Work out the finished part from the listing and answer in its coordinate system (mm). Coordinates: 2 decimals unless noted, no trailing zeros. Order: outer loops, then holes, each group sorted by start corner. A loop starts at its lowest first (then second) coordinate and runs counter-clockwise, first axis right, second up. Notation, with made-up numbers: (5.25, 61.25) -> (60.25, 61.25) arc R34 ccw to (60.25, 100.25) -> close; hole circle Ø3 at (0.25, 58.5). An arc over 180 degrees is marked (long way). Use one line per item in the form item = value.
from build123d import *

# Parameters (mm, degrees)
SKETCH_1_W      = 63
SKETCH_1_H      = 42
SKETCH_1_R      = 4.5
SKETCH_1_W_2    = 10
SKETCH_1_W_3    = 42
SKETCH_1_R_2    = 1.6
SKETCH_1_W_4    = 5
EXTRUDE_1_DEPTH = 6
FILLET_1_R      = 5


with BuildPart() as part:
    # 草图1 → 凸台-拉伸1 (new body)
    # profile 1 of 7: a face of its own
    with BuildSketch(Plane.XY):
        with Locations((-109.5, 0)):
            Rectangle(SKETCH_1_W, SKETCH_1_H)
        with Locations((-132, 0)):
            Circle(SKETCH_1_R, mode=Mode.SUBTRACT)
    # profile 2 of 7: a face of its own
    with BuildSketch(Plane.XY):
        with BuildLine():
            Line((-73, 21), (-78, 21))
            Line((-78, 21), (-78, -21))
            Line((-78, -21), (-73, -21))
            Line((-73, -21), (-73, -17.019868415))
            ThreePointArc((-73, -17.019868415), (-74.1, -15.5), (-73, -13.980131585))
            Line((-73, -13.980131585), (-73, 13.980131585))
            ThreePointArc((-73, 13.980131585), (-74.1, 15.5), (-73, 17.019868415))
            Line((-73, 17.019868415), (-73, 21))
        make_face()
    # profile 3 of 7: a face of its own
    with BuildSketch(Plane.XY):
        with BuildLine():
            Line((-36, 21), (-73, 21))
            Line((-73, 21), (-73, 17.019868415))
            ThreePointArc((-73, 17.019868415), (-72.753190181, 17.079840097), (-72.5, 17.1))
            Line((-72.5, 17.1), (-67.5, 17.1))
            ThreePointArc((-67.5, 17.1), (-65.9, 15.5), (-67.5, 13.9))
            Line((-67.5, 13.9), (-72.5, 13.9))
            ThreePointArc((-72.5, 13.9), (-72.753190181, 13.920159903), (-73, 13.980131585))
            Line((-73, 13.980131585), (-73, -13.980131585))
            ThreePointArc((-73, -13.980131585), (-72.753190181, -13.920159903), (-72.5, -13.9))
            Line((-72.5, -13.9), (-67.5, -13.9))
            ThreePointArc((-67.5, -13.9), (-65.9, -15.5), (-67.5, -17.1))
            Line((-67.5, -17.1), (-72.5, -17.1))
            ThreePointArc((-72.5, -17.1), (-72.753190181, -17.079840097), (-73, -17.019868415))
            Line((-73, -17.019868415), (-73, -21))
            Line((-73, -21), (-36, -21))
            Line((-36, -21), (-36, -17.019868415))
            ThreePointArc((-36, -17.019868415), (-36.246809819, -17.079840097), (-36.5, -17.1))
            Line((-36.5, -17.1), (-41.5, -17.1))
            ThreePointArc((-41.5, -17.1), (-43.1, -15.5), (-41.5, -13.9))
            Line((-41.5, -13.9), (-36.5, -13.9))
            ThreePointArc((-36.5, -13.9), (-36.246809819, -13.920159903), (-36, -13.980131585))
            Line((-36, -13.980131585), (-36, 13.980131585))
            ThreePointArc((-36, 13.980131585), (-36.246809819, 13.920159903), (-36.5, 13.9))
            Line((-36.5, 13.9), (-41.5, 13.9))
            ThreePointArc((-41.5, 13.9), (-43.1, 15.5), (-41.5, 17.1))
            Line((-41.5, 17.1), (-36.5, 17.1))
            ThreePointArc((-36.5, 17.1), (-36.246809819, 17.079840097), (-36, 17.019868415))
            Line((-36, 17.019868415), (-36, 21))
        make_face()
        with BuildLine():
            ThreePointArc((-57, -2.5), (-59.5, 0), (-57, 2.5))
            Line((-57, 2.5), (-52, 2.5))
            ThreePointArc((-52, 2.5), (-49.5, 0), (-52, -2.5))
            Line((-52, -2.5), (-57, -2.5))
        make_face(mode=Mode.SUBTRACT)
    # profile 4 of 7: a face of its own
    with BuildSketch(Plane.XY):
        with BuildLine():
            Line((-31, 21), (-36, 21))
            Line((-36, 21), (-36, 17.019868415))
            ThreePointArc((-36, 17.019868415), (-34.9, 15.5), (-36, 13.980131585))
            Line((-36, 13.980131585), (-36, -13.980131585))
            ThreePointArc((-36, -13.980131585), (-34.9, -15.5), (-36, -17.019868415))
            Line((-36, -17.019868415), (-36, -21))
            Line((-36, -21), (-31, -21))
            Line((-31, -21), (-31, 21))
        make_face()
    # profile 5 of 7: a face of its own
    with BuildSketch(Plane.XY):
        with Locations((-26, 0)):
            Rectangle(SKETCH_1_W_2, SKETCH_1_H)
    # profile 6 of 7: a face of its own
    with BuildSketch(Plane.XY):
        Rectangle(SKETCH_1_W_3, SKETCH_1_H)
        with Locations((15.5, -15.5)):
            Circle(SKETCH_1_R_2, mode=Mode.SUBTRACT)
        with Locations((-15.5, -15.5)):
            Circle(SKETCH_1_R_2, mode=Mode.SUBTRACT)
        with Locations((15.5, 15.5)):
            Circle(SKETCH_1_R_2, mode=Mode.SUBTRACT)
        with Locations((-15.5, 15.5)):
            Circle(SKETCH_1_R_2, mode=Mode.SUBTRACT)
        Circle(SKETCH_1_R_2, mode=Mode.SUBTRACT)
    # profile 7 of 7: a face of its own
    with BuildSketch(Plane.XY):
        with Locations((-143.5, 0)):
            Rectangle(SKETCH_1_W_4, SKETCH_1_H)
    extrude(amount=EXTRUDE_1_DEPTH)

    # 圆角1
    fillet_1_edges = [part.edges().sort_by_distance(p)[0] for p in [
        (-146, 21, 3),
        (-146, -21, 3),
    ]]
    fillet(fillet_1_edges, radius=FILLET_1_R)


solid = part.part
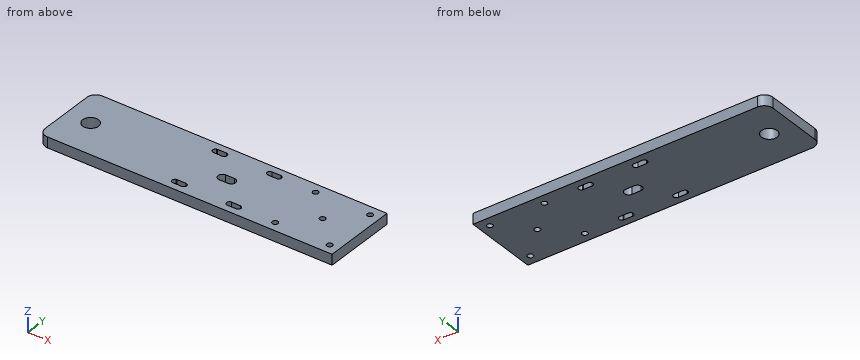
(1) This flat-tipped pin is pushed along its axis until it touches: P1, Ø5, axis at x = 15.5, y = -15.5, coming from the +Z side. Where does it stop, or does it pass through?
Data:
P1 = 6
(2) Straight lines are drawn through the part: line 1 along Y through (x, z) = (-73, 5.3); line 2 along Y through (x, z) = (-15.5, 2.5); line 3 along Y through (x, z) = (-132, 2.6). For each, find the intervals that lie inside material, in ascending order.
Data:
line_1 = -21 to -17.02, -13.98 to 13.98, 17.02 to 21
line_2 = -21 to -17.1, -13.9 to 13.9, 17.1 to 21
line_3 = -21 to -4.5, 4.5 to 21
(3) Section C-C on z = 1.3 is taken. Count the separate pieces of the cut face and the enclosed holes in it, plus the area to 3 significant figures.
Data:
separate_pieces = 1
enclosed_holes = 11
area = 6,760 mm²
(4) Section A-A on x = -132 is taken. Write down the section's boundary in (y, z), plus the area to 3 significant figures.
Data:
outline = (-21, 0) -> (-4.5, 0) -> (-4.5, 6) -> (-21, 6) -> close; (4.5, 0) -> (21, 0) -> (21, 6) -> (4.5, 6) -> close
area = 198 mm²
(5) Section B-B on x = -15.5 is taken. Write down the section's boundary in (y, z), plus the area to 3 significant figures.
Data:
outline = (-21, 0) -> (-17.1, 0) -> (-17.1, 6) -> (-21, 6) -> close; (-13.9, 0) -> (13.9, 0) -> (13.9, 6) -> (-13.9, 6) -> close; (17.1, 0) -> (21, 0) -> (21, 6) -> (17.1, 6) -> close
area = 214 mm²
